Work out the finished part from the listing and answer in its coordinate system (mm). Round coordinates to 2 decimals unless told otherwise and drop trailing zeros. Write each loop counter-clockwise with the first axis right and the second up, starting at its lowest first coordinate (ties: lowest second). Pieces come first, ordered by that corner, then holes.
1. Flat-ended cylindrical pins translate along their axes: pin 1 Ø24 at (x, z) = (17.5, 19.5) entering from +Y; pin 2 Ø6 at (x, y) = (-22, 10) entering from +Z. Find the tip coordinate at first contact, or state that the pin passes through.
2. Find section B-B (x = 0). Write down the section's boundary in (y, z), and give its area (3 significant figures).
3. Find section D-D (y = 23). Write down the section's boundary in (x, z).
4. Determine the mould class of faces 1 (the face through (-0.867, 17.332, 3.905)), 2 (the face through (8, 5.5, -1)), 3 (the face through (6.659, 2.788, -27.055)) for opening direction Z: pulls with the +Z half, pulls with the -Z half, needs draft (parallel to the pull), parting line crosses it, or undercut.
5. Find section C-C (x = 30). Write down the section's boundary in (y, z), and give its area (3 significant figures).
6. Straight lines are drawn through the part: probe 1 along X at (y, z) = (3.3, 0); probe 2 along Y at (x, z) = (-13, -23); probe 3 along Z at (x, y) = (10.5, 2.75). For each, find the intervals that lie inside material, in ascending order.
7. Find section A-A (z = 0). Write down the section's boundary in (x, y), and give its area (3 significant figures).
```python
from build123d import *

# Parameters (mm, degrees)
SKETCH1_R           = 40
BOSS_EXTRUDE1_DEPTH = 5.5
SKETCH2_R           = 3
CUT_EXTRUDE1_DEPTH  = 6.5
CIRPATTERN1_COUNT   = 5
SKETCH3_R           = 4
BOSS_EXTRUDE2_DEPTH = 24


with BuildPart() as part:
    # Sketch1 → Boss-Extrude1 (new body)
    with BuildSketch(Plane(origin=(0, 0, 0), x_dir=(1, 0, 0), z_dir=(0, 1, 0))):
        Circle(SKETCH1_R)
    extrude(amount=BOSS_EXTRUDE1_DEPTH)

    # Sketch2 → Cut-Extrude1 (cut, through all)
    with BuildSketch(Plane(origin=(0, 5.5, 0), x_dir=(1, 0, 0), z_dir=(0, 1, 0))):
        with Locations((30, 0)):
            Circle(SKETCH2_R)
    cut_extrude1 = extrude(amount=-CUT_EXTRUDE1_DEPTH, mode=Mode.SUBTRACT)

    # CirPattern1: Cut-Extrude1 ×5 about axis
    cirpattern1_axis = Axis((0, 0, 0), (0, 1, 0))
    for i in range(1, CIRPATTERN1_COUNT):
        add(cut_extrude1.rotate(cirpattern1_axis, i * 360 / CIRPATTERN1_COUNT), mode=Mode.SUBTRACT)

    # Sketch3 → Boss-Extrude2 (add)
    with BuildSketch(Plane(origin=(0, 5.5, 0), x_dir=(1, 0, 0), z_dir=(0, 1, 0))):
        Circle(SKETCH3_R)
    extrude(amount=BOSS_EXTRUDE2_DEPTH)


solid = part.part
```
Worked answers:
1. pin 1: stops at y = 5.5
1. pin 2: passes through
2. outline: (0, -40) - (5.5, -40) - (5.5, -4) - (29.5, -4) - (29.5, 4) - (5.5, 4) - (5.5, 40) - (0, 40) - close
2. area: 632 mm2
3. outline: circle Ø8 at (0, 0)
4. face 1: parting line crosses it
4. face 2: needs draft
4. face 3: undercut
5. outline: (0, -26.46) - (5.5, -26.46) - (5.5, -3) - (0, -3) - close; (0, 3) - (5.5, 3) - (5.5, 26.46) - (0, 26.46) - close
5. area: 258 mm2
6. probe 1: x = -40 to 27, 33 to 40
6. probe 2: y = 0 to 5.5
6. probe 3: z = -38.6 to -31.27, -25.8 to 25.8, 31.27 to 38.6
7. outline: (-40, 0) - (27, 0) - (27, 5.5) - (4, 5.5) - (4, 29.5) - (-4, 29.5) - (-4, 5.5) - (-40, 5.5) - close; (33, 0) - (40, 0) - (40, 5.5) - (33, 5.5) - close
7. area: 599 mm2
